from build123d import *

# Parameters (mm, degrees)
SKETCH1_W                        = 160
SKETCH1_H                        = 45
EXTRUDE1_DEPTH                   = 13
SKETCH2_W                        = 100
SKETCH2_H                        = 45
EXTRUDE2_DEPTH                   = 12
SKETCH3_W                        = 70
SKETCH3_H                        = 12
EXTRUDE3_DEPTH                   = 26
FILLET1_R                        = 2.5
F_4_40_TAPPED_HOLE1_AT_2_COUNT   = 2
F_4_40_TAPPED_HOLE1_AT_2_PITCH   = 49.648766349
F_4_40_TAPPED_HOLE1_AT_3_COUNT   = 2
F_4_40_TAPPED_HOLE1_AT_3_PITCH   = 56.435804238
F_4_40_TAPPED_HOLE1_AT_4_COUNT   = 2
F_4_40_TAPPED_HOLE1_AT_4_PITCH   = 36
F_1_4_20_TAPPED_HOLE1_AT_2_COUNT = 2
F_1_4_20_TAPPED_HOLE1_AT_2_PITCH = 25
SKETCH7_R                        = 0.75
EXTRUDE4_DEPTH                   = 7


with BuildPart() as part:
    # Sketch1 → Extrude1 (new body)
    with BuildSketch(Plane(origin=(0, 0, 0), x_dir=(1, 0, 0), z_dir=(0, 1, 0))):
        Rectangle(SKETCH1_W, SKETCH1_H)
    extrude(amount=EXTRUDE1_DEPTH)

    # Sketch2 → Extrude2 (add)
    with BuildSketch(Plane.XZ):
        Rectangle(SKETCH2_W, SKETCH2_H)
    extrude(amount=EXTRUDE2_DEPTH)

    # Sketch3 → Extrude3 (cut, through all)
    with BuildSketch(Plane(origin=(0, 13, 0), x_dir=(1, 0, 0), z_dir=(0, 1, 0))):
        with Locations((0, -1.5)):
            Rectangle(SKETCH3_W, SKETCH3_H)
    extrude(amount=-EXTRUDE3_DEPTH, mode=Mode.SUBTRACT)

    # Fillet1
    fillet1_edges = [part.edges().sort_by_distance(p)[0] for p in [
        (-35, 0.5, 7.5),
        (-35, 0.5, -4.5),
        (35, 0.5, -4.5),
        (35, 0.5, 7.5),
    ]]
    fillet(fillet1_edges, radius=FILLET1_R)

    # Sketch5 → #4-40 Tapped Hole1 (revolve, cut)
    with BuildSketch(Plane(origin=(-72.77, 13, 19.5), x_dir=(0, 0, 1), z_dir=(1, 0, 0))):
        Polygon((0, 0), (0, 26.053752758), (1.1303, 25.3746), (1.1303, 5.6896), (1.4224, 5.6896), (1.4224, 0), align=None)
    f_4_40_tapped_hole1 = revolve(axis=Axis((-72.77, 19.35, 19.5), (0, -1, 0)), mode=Mode.SUBTRACT)

    # #4-40 Tapped Hole1 at 2: #4-40 Tapped Hole1 ×2
    with Locations(*[Vector(0.986932881, 0, -0.161131899) * (i * F_4_40_TAPPED_HOLE1_AT_2_PITCH) for i in range(1, F_4_40_TAPPED_HOLE1_AT_2_COUNT)]):
        add(f_4_40_tapped_hole1, mode=Mode.SUBTRACT)

    # #4-40 Tapped Hole1 at 3: #4-40 Tapped Hole1 ×2
    with Locations(*[Vector(0.868243142, 0, -0.496138938) * (i * F_4_40_TAPPED_HOLE1_AT_3_PITCH) for i in range(1, F_4_40_TAPPED_HOLE1_AT_3_COUNT)]):
        add(f_4_40_tapped_hole1, mode=Mode.SUBTRACT)

    # #4-40 Tapped Hole1 at 4: #4-40 Tapped Hole1 ×2
    with Locations(*[(0, 0, -i * F_4_40_TAPPED_HOLE1_AT_4_PITCH) for i in range(1, F_4_40_TAPPED_HOLE1_AT_4_COUNT)]):
        add(f_4_40_tapped_hole1, mode=Mode.SUBTRACT)

    # Mirror1: #4-40 Tapped Hole1 across plane
    add(f_4_40_tapped_hole1.mirror(Plane(origin=(0, 0, 0), x_dir=(0, 0, 1), z_dir=(1, 0, 0))), mode=Mode.SUBTRACT)

    # Mirror1 copy 1 sketch → Mirror1 copy 1 (revolve, cut)
    with BuildSketch(Plane(origin=(23.77, 13, 11.5), x_dir=(0, 0, 1), z_dir=(-1, 0, 0))):
        Polygon((0, 0), (0, -26.053752758), (1.1303, -25.3746), (1.1303, -5.6896), (1.4224, -5.6896), (1.4224, 0), align=None)
    revolve(axis=Axis((23.77, 19.35, 11.5), (0, 1, 0)), mode=Mode.SUBTRACT)

    # Mirror1 copy 2 sketch → Mirror1 copy 2 (revolve, cut)
    with BuildSketch(Plane(origin=(23.77, 13, -8.5), x_dir=(0, 0, 1), z_dir=(-1, 0, 0))):
        Polygon((0, 0), (0, -26.053752758), (1.1303, -25.3746), (1.1303, -5.6896), (1.4224, -5.6896), (1.4224, 0), align=None)
    revolve(axis=Axis((23.77, 19.35, -8.5), (0, 1, 0)), mode=Mode.SUBTRACT)

    # Mirror1 copy 3 sketch → Mirror1 copy 3 (revolve, cut)
    with BuildSketch(Plane(origin=(72.77, 13, -16.5), x_dir=(0, 0, 1), z_dir=(-1, 0, 0))):
        Polygon((0, 0), (0, -26.053752758), (1.1303, -25.3746), (1.1303, -5.6896), (1.4224, -5.6896), (1.4224, 0), align=None)
    revolve(axis=Axis((72.77, 19.35, -16.5), (0, 1, 0)), mode=Mode.SUBTRACT)

    # Sketch6 → 1/4-20 Tapped Hole1 (revolve, cut)
    with BuildSketch(Plane(origin=(50, -7, -14.5), x_dir=(0, 0, -1), z_dir=(0, 1, 0))):
        Polygon((0, 0), (0, 21.533827702), (2.5527, 20.0000108), (2.5527, 12.7), (3.175, 12.7), (3.175, 0), align=None)
    f_1_4_20_tapped_hole1 = revolve(axis=Axis((56.35, -7, -14.5), (-1, 0, 0)), mode=Mode.SUBTRACT)

    # 1/4-20 Tapped Hole1 at 2: 1/4-20 Tapped Hole1 ×2
    with Locations(*[(0, 0, i * F_1_4_20_TAPPED_HOLE1_AT_2_PITCH) for i in range(1, F_1_4_20_TAPPED_HOLE1_AT_2_COUNT)]):
        add(f_1_4_20_tapped_hole1, mode=Mode.SUBTRACT)

    # Sketch7 → Extrude4 (cut)
    with BuildSketch(Plane.XZ.offset(12)):
        with Locations(Location((31, -14.5, 0), (0, 0, 270))):  # turned: the seam where the file's is
            Circle(SKETCH7_R)
        with Locations(Location((31, 10.5, 0), (0, 0, 270))):  # turned: the seam where the file's is
            Circle(SKETCH7_R)
    extrude4 = extrude(amount=-EXTRUDE4_DEPTH, mode=Mode.SUBTRACT)

    # Mirror2: Extrude4, 1/4-20 Tapped Hole1 across plane
    add(extrude4.mirror(Plane(origin=(0, 0, 0), x_dir=(0, 0, 1), z_dir=(1, 0, 0))), mode=Mode.SUBTRACT)
    add(f_1_4_20_tapped_hole1.mirror(Plane(origin=(0, 0, 0), x_dir=(0, 0, 1), z_dir=(1, 0, 0))), mode=Mode.SUBTRACT)

    # Mirror2 copy 1 sketch → Mirror2 copy 1 (revolve, cut)
    with BuildSketch(Plane(origin=(-50, -7, 10.5), x_dir=(0, 0, -1), z_dir=(0, 1, 0))):
        Polygon((0, 0), (0, -21.533827702), (2.5527, -20.0000108), (2.5527, -12.7), (3.175, -12.7), (3.175, 0), align=None)
    revolve(axis=Axis((-56.35, -7, 10.5), (-1, 0, 0)), mode=Mode.SUBTRACT)

    # Sketch8 → #4-40 Tapped Hole2 (revolve, cut)
    with BuildSketch(Plane(origin=(15, -9, -22.5), x_dir=(0, 1, 0), z_dir=(1, 0, 0))):
        Polygon((0, 0), (0, 20.973752758), (1.1303, 20.2946), (1.1303, 8.2296), (1.4224, 8.2296), (1.4224, 0), align=None)
    f_4_40_tapped_hole2 = revolve(axis=Axis((15, -9, -28.85), (0, 0, 1)), mode=Mode.SUBTRACT)

    # Mirror3: #4-40 Tapped Hole2 across plane
    add(f_4_40_tapped_hole2.mirror(Plane(origin=(0, 0, 0), x_dir=(0, 0, 1), z_dir=(1, 0, 0))), mode=Mode.SUBTRACT)


solid = part.part
Verification items for the finished model (mm, model axes). A direction names the side the tool comes from. Give positions to 0.01 mm unless a question says otherwise; leave off trailing zeros. Write each loop counter-clockwise with the first axis right and the second up, starting at its lowest first coordinate (ties: lowest second). Pieces come first, ordered by that corner, then holes. Notation, with made-up numbers: (57.5, -32) - (106.5, -32) arc R10 ccw to (106.5, -24) - close; hole circle Ø7 at (30.5, 5.25). An arc over 180 degrees is marked (long way). Answer as CSV lines item,"result". Start each with the question number.
1. Draft check along X on faces 5 (the face through (0, 1, -4.5)), 6 (the face through (28.73, -6.73, -14.15)), 7 (the face through (43.74, -7.95, -17.53)), 8 (the face through (-50, -6, 0)). Enter one of: pulls with the +X half, pulls with the -X half, needs draft (parallel to the pull), parting line crosses it, or undercut.
2. Thickness scan on line 1 (X direction, y = 3, z = 19.5); line 2 (X direction, y = 8.9, z = -16.5); line 3 (X direction, y = 9, z = 4.5). Record the ranges inside material, lowest first.
3. Sectioned sample at D-D (x = -43). Record the boundary of the cut face in (y, z) (3 decimals).
4. Set-up check for faces 1 (the face through (43.74, -10.15, 10.91)), 2 (the face through (71.904, 10.195, 18.371)), 3 (the face through (65, 0, 0)), 4 (the face through (-33.701, -4.735, 9.322)): record each of +Z, -Z, +X, -X, +Y, -Y from which the full face is reachable in a straight line by a thin tool's end or side.
5. Depth check by flat-ended pin: pin 1 (24 mm diameter, centred on x = -66, z = 3.5, fed in from -Y); pin 2 (2.5 mm diameter, centred on x = -14.5, y = -8.5, fed in from -Z); pin 3 (2.5 mm diameter, centred on x = -15, y = -9, fed in from -Z); pin 4 (5 mm diameter, centred on y = -8.5, z = 9, fed in from +X). Enter the tip coordinate at first touch or a pass-through.
6. Sectioned sample at C-C (x = -7). Record the boundary of the cut face in (y, z), then the cut area to 3 significant figures.
7. Sectioned sample at B-B (y = 9.25). Count the separate pieces of the cut face and the enclosed holes in it, then the cut area to 3 significant figures.
8. Sectioned sample at A-A (z = 0). Record the boundary of the cut face in (x, y), then the cut area to 3 significant figures.
Derived:
1,face 5,"undercut"
1,face 6,"pulls with the +X half"
1,face 7,"needs draft"
1,face 8,"pulls with the -X half"
2,line 1,"-80 to -73.9, -71.64 to 71.64, 73.9 to 80"
2,line 2,"-80 to -74.19, -71.35 to 71.35, 74.19 to 80"
2,line 3,"-80 to -35, 35 to 80"
3,outline,"(-12, -22.5) - (13, -22.5) - (13, 22.5) - (-12, 22.5) - close; hole circle Ø6.35 at (-7, -14.5); hole circle Ø6.35 at (-7, 10.5)"
4,face 1,"+X"
4,face 2,"+Y"
4,face 3,"+Z, -Z, +X, -Y"
4,face 4,"-X"
5,pin 1,"y = 0"
5,pin 2,"z = -22.5"
5,pin 3,"z = -14.27"
5,pin 4,"x = 50"
6,outline,"(-12, -22.5) - (13, -22.5) - (13, -4.5) - (-12, -4.5) - close; (-12, 7.5) - (13, 7.5) - (13, 22.5) - (-12, 22.5) - close"
6,area,"825 mm²"
7,separate pieces,"1"
7,enclosed holes,"9"
7,area,"6,310 mm²"
8,outline,"(-80, 0) - (-50, 0) - (-50, -12) - (-35, -12) - (-35, 13) - (-80, 13) - close; (35, -12) - (50, -12) - (50, 0) - (80, 0) - (80, 13) - (35, 13) - close"
8,area,"1,530 mm²"
